Design review of the part built by this model. Coordinates are the model's own, in mm. A direction names the side the tool comes from. Coordinates: 2 decimals unless noted, no trailing zeros. Write each loop counter-clockwise with the first axis right and the second up, starting at its lowest first coordinate (ties: lowest second). Pieces come first, ordered by that corner, then holes. Notation, with made-up numbers: (89, -39.5) - (126, -39.5) arc R6 cw to (126, -35.5) - close; hole circle Ø11 at (35, -16.5). An arc over 180 degrees is marked (long way). Answer as CSV lines item,"result". Start each with the question number.
Q1. For line 1 along Y through (x, z) = (6.5, -47); line 2 along Z through (x, y) = (7.5, -49.5); line 3 along Z through (x, y) = (9, 28), list the stretches that pass through material, from the lowest coordinate up. Write a range as [from, to].
Q2. We need section C-C (y = 29). Write out the cut boundary in (x, z), plus the area to 3 significant figures.
Q3. We need section A-A (z = -97.5). Write out the cut boundary in (x, y).
Q4. Machinability: for faces 1 (the face through (5, -50, -100)), 2 (the face through (5, 25, -140)), 3 (the face through (5, -49, -135)), 4 (the face through (5, -48, 135)), 5 (the face through (5, 25, 140)), which of the approach directions +Z, -Z, +X, -X, +Y, -Y give a long, thin tool a straight path to every point of the face, cutting with its end or side? Answer none if there is none.
Q5. We need section B-B (x = 3.75). Write out the cut boundary in (y, z).
Q6. Mouldability with a two-part tool opening along Z and no side actions: class faces 6 (the face through (5, 45, 2)), 7 (the face through (5, -50, 100)), 8 (the face through (5, -5, -145)) as pulls with the +Z half, pulls with the -Z half, needs draft (parallel to the pull), parting line crosses it, or undercut.
Q7. Clearance check with flat-ended pins moving along their axes: pin 1 (3 mm diameter, centred on x = 7, y = -52, fed in from -Z); pin 2 (12 mm diameter, centred on y = -17.5, z = -69.5, fed in from -X); pin 3 (3 mm diameter, centred on x = 7, z = 142.5, fed in from +Y); pin 4 (5 mm diameter, centred on x = 4.5, y = -46, fed in from +Z). State where each tip first meets the part, or that it passes through.
Autodesk Inventor part; units mm, degrees
ref_plane "YZ Plane" through (0, 0, 0) normal (1, 0, 0) x (0, 1, 0)
ref_plane "XZ Plane" through (0, 0, 0) normal (0, 1, 0) x (-1, 0, 0)
ref_plane "XY Plane" through (0, 0, 0) normal (0, 0, 1) x (1, 0, 0)
sketch "Sketch1" plane through (0, 0, 0) normal (1, 0, 0) x (0, 1, 0)
  line L0 (-45, 135) -> (45, 135)
  line L1 (45, 135) -> (45, -135)
  line L2 (45, -135) -> (-45, -135)
  line L3 (-45, -135) -> (-45, 135)
  line L4 (-45, 135) -> (45, -135) construction
  line L5 (45, 135) -> (-45, -135) construction
  point P0 (0, 0)
  dimension "d0" = 90
  dimension "d1" = 270
extrude "Extrusion1" add sketch "Sketch1" along normal blind 10
sketch "Sketch2" plane through (0, 0, 0) normal (-1, 0, 0) x (0, 0, 1)
  line L0 (-135, -45) -> (-135, 45)
  line L1 (135, -45) -> (-135, -45)
  line L2 (135, 45) -> (135, -45)
  line L3 (-135, 45) -> (135, 45)
  line L4 (0, 45) -> (0, -5)
  line L5 (145, 25) -> (-145, 25)
  line L6 (-145, 25) -> (-145, -35)
  line L7 (-145, -35) -> (145, -35)
  line L8 (145, -35) -> (145, 25)
  line L9 (145, 25) -> (-145, -35) construction
  line L10 (-145, 25) -> (145, -35) construction
  point P0 (-135, -35)
  point P1 (-135, 25)
  point P2 (135, 25)
  point P3 (135, -35)
  dimension "d8" = 90
  dimension "d9" = 50
  dimension "d10" = 60
  dimension "d11" = 290
  dimension "d12" = 270
extrude "Extrusion2" add sketch "Sketch2" against normal blind 10 contours L7 L6 L5 L0 | L2 L5 L8 L7
sketch "Sketch3" plane through (10, 0, 0) normal (1, 0, 0) x (0, 0, -1)
  line L0 (135, -45) -> (135, -35)
  line L1 (135, -35) -> (145, -35)
  line L2 (145, -35) -> (145, 25)
  line L3 (145, 25) -> (135, 25)
  line L4 (135, 25) -> (135, 45)
  line L5 (135, 45) -> (-135, 45)
  line L6 (-135, 45) -> (-135, 25)
  line L7 (-135, 25) -> (-145, 25)
  line L8 (-145, 25) -> (-145, -35)
  line L9 (-145, -35) -> (-135, -35)
  line L10 (-135, -35) -> (-135, -45)
  line L11 (-135, -45) -> (135, -45)
  line L12 (135, -20) -> (-135, -20)
  line L13 (-135, -20) -> (-135, -70)
  line L14 (-135, -70) -> (135, -70)
  line L15 (135, -70) -> (135, -20)
  line L16 (135, -20) -> (-135, -70) construction
  line L17 (-135, -20) -> (135, -70) construction
  line L18 (100, -35) -> (-100, -35)
  line L19 (-100, -35) -> (-100, -55)
  line L20 (-100, -55) -> (100, -55)
  line L21 (100, -55) -> (100, -35)
  line L22 (100, -35) -> (-100, -55) construction
  line L23 (-100, -35) -> (100, -55) construction
  point P0 (0, 0)
  point P1 (0, -45)
  point P2 (100, -45)
  point P3 (-100, -45)
  dimension "d13" = 25
  dimension "d14" = 200
  dimension "d15" = 10
extrude "Extrusion3" add sketch "Sketch3" against normal blind 10 contours L15 L14 L13 L11 L19 L20 L21
chamfer "Chamfer1" distance 8.25 angle 45 2 edges at (5, -70, 135) (5, -70, -135)
properties part number "03_Tam_mat_truoc" material "Stainless Steel, Austenitic"
Results list:
1,line 1,"y = [-70, -55], [-45, 45]"
1,line 2,"z = [-135, -100], [100, 135]"
1,line 3,"z = [-135, 135]"
2,outline,"(0, -135) - (10, -135) - (10, 135) - (0, 135) - close"
2,area,"2,700 mm2"
3,outline,"(0, -70) - (10, -70) - (10, -55) - (0, -55) - close; (0, -45) - (10, -45) - (10, 45) - (0, 45) - close"
4,face 1,"+X, -X"
4,face 2,"-Z, +X, -X, +Y"
4,face 3,"-Z, +X, -X, -Y"
4,face 4,"+Z, +X, -X, -Y"
4,face 5,"+Z, +X, -X, +Y"
5,outline,"(-70, -126.75) - (-61.75, -135) - (-35, -135) - (-35, -145) - (25, -145) - (25, -135) - (45, -135) - (45, 135) - (25, 135) - (25, 145) - (-35, 145) - (-35, 135) - (-61.75, 135) - (-70, 126.75) - close; hole (-55, -100) - (-45, -100) - (-45, 100) - (-55, 100) - close"
6,face 6,"needs draft"
6,face 7,"undercut"
6,face 8,"pulls with the -Z half"
7,pin 1,"stops at z = -135"
7,pin 2,"stops at x = 0"
7,pin 3,"stops at y = 25"
7,pin 4,"stops at z = 135"
